Can you work these out from the model? Positions are in its coordinate system, mm. Face numbers are marked on the shaded views. A direction names the side the tool comes from. Give positions to 0.01 mm unless a question says otherwise; leave off trailing zeros. Write each loop counter-clockwise with the first axis right and the second up, starting at its lowest first coordinate (ties: lowest second). Pieces come first, ordered by that corner, then holes.
from build123d import *

# Parameters (mm, degrees)
SKETCH_1_W          = 40
SKETCH_1_H          = 20
EXTRUDE_1_DEPTH     = 3.5
SKETCH_2_W          = 40
SKETCH_2_H          = 20
SKETCH_2_R          = 5.25
EXTRUDE_2_DEPTH     = 1.5
EXTRUDE_3_DEPTH     = 8
SKETCH_4_W          = 40
SKETCH_4_H          = 12
SKETCH_4_R          = 3.5
EXTRUDE_4_DEPTH     = 5
FILLET_1_R          = 1.5
SKETCH_5_R          = 1.75
CUT_EXTRUDE_1_DEPTH = 5
CUT_EXTRUDE_2_DEPTH = 3
CUT_EXTRUDE_3_DEPTH = 3.5
CUT_EXTRUDE_START   = -3.5
SKETCH_8_R          = 5.45
SKETCH_8_R_2        = 5.25
CUT_EXTRUDE_4_DEPTH = 3.5


with BuildPart() as part:
    # 草图1 → 凸台-拉伸1 (new body)
    with BuildSketch(Plane.XY):
        Rectangle(SKETCH_1_W, SKETCH_1_H)
        with BuildLine():
            Line((-9.5, -5.75), (9.5, -5.75))
            ThreePointArc((9.5, -5.75), (11, 0), (9.5, 5.75))
            Line((9.5, 5.75), (-9.5, 5.75))
            ThreePointArc((-9.5, 5.75), (-11, 0), (-9.5, -5.75))
        make_face(mode=Mode.SUBTRACT)
    extrude(amount=EXTRUDE_1_DEPTH)

    # 草图2 → 凸台-拉伸2 (add)
    with BuildSketch(Plane.XY.offset(3.5)):
        Rectangle(SKETCH_2_W, SKETCH_2_H)
        Circle(SKETCH_2_R, mode=Mode.SUBTRACT)
    extrude(amount=EXTRUDE_2_DEPTH)

    # 草图3 → 凸台-拉伸3 (add)
    with BuildSketch(Plane.XY.offset(5)):
        Polygon((-16.560660172, 5.5), (-18.2, 5.5), (-18.2, 3.1), (-20, 3.1), (-20, -3.1), (-18.2, -3.1), (-18.2, -5.5), (-16.560660172, -5.5), (-13.9, -2.839339828), (-13.9, 2.839339828), align=None)
        Polygon((18.2, 3.1), (20, 3.1), (20, -3.1), (18.2, -3.1), (18.2, -5.5), (16.560660172, -5.5), (13.9, -2.839339828), (13.9, 2.839339828), (16.560660172, 5.5), (18.2, 5.5), align=None)
    extrude(amount=-EXTRUDE_3_DEPTH)

    # 草图4 → 凸台-拉伸4 (add)
    with BuildSketch(Plane.XY.offset(5)):
        with Locations((0, 16)):
            Rectangle(SKETCH_4_W, SKETCH_4_H)
        with Locations((-10, 14.64)):
            Circle(SKETCH_4_R, mode=Mode.SUBTRACT)
        with Locations((10, 14.64)):
            Circle(SKETCH_4_R, mode=Mode.SUBTRACT)
    extrude(amount=-EXTRUDE_4_DEPTH)

    # 圆角1
    fillet_1_edges = [part.edges().sort_by_distance(p)[0] for p in [
        (20, 22, 2.5),
        (-20, 22, 2.5),
        (20, -10, 2.5),
        (-20, -10, 2.5),
    ]]
    fillet(fillet_1_edges, radius=FILLET_1_R)

    # 草图5 → 切除-拉伸1 (cut)
    with BuildSketch(Plane.XY.offset(5)):
        with Locations((0, 14.64)):
            Circle(SKETCH_5_R)
    extrude(amount=-CUT_EXTRUDE_1_DEPTH, mode=Mode.SUBTRACT)

    # 草图6 → 切除-拉伸2 (cut)
    with BuildSketch(Plane(origin=(0, 0, -3), x_dir=(-1, 0, 0), z_dir=(0, 0, -1))):
        Polygon((-18.2, 5.5), (-18.2, 3.1), (-20, 3.1), (-20, 2.6), (-19.5, 2.6), (-17.7, 2.6), (-17.7, 5), (-16.767766953, 5), (-14.4, 2.632233047), (-14.4, -2.632233047), (-16.767766953, -5), (-17.7, -5), (-17.7, -2.6), (-19.5, -2.6), (-20, -2.6), (-20, -3.1), (-18.2, -3.1), (-18.2, -5.5), (-16.560660172, -5.5), (-13.9, -2.839339828), (-13.9, 2.839339828), (-16.560660172, 5.5), align=None)
        Polygon((18.2, -5.5), (18.2, -3.1), (20, -3.1), (20, -2.6), (19.5, -2.6), (17.7, -2.6), (17.7, -5), (16.767766953, -5), (14.4, -2.632233047), (14.4, 2.632233047), (16.767766953, 5), (17.7, 5), (17.7, 2.6), (19.5, 2.6), (20, 2.6), (20, 3.1), (18.2, 3.1), (18.2, 5.5), (16.560660172, 5.5), (13.9, 2.839339828), (13.9, -2.839339828), (16.560660172, -5.5), align=None)
    extrude(amount=-CUT_EXTRUDE_2_DEPTH, mode=Mode.SUBTRACT)

    # 草图7 → 切除-拉伸3 (cut)
    with BuildSketch(Plane(origin=(0, 0, 0), x_dir=(-1, 0, 0), z_dir=(0, 0, -1))):
        with BuildLine():
            Line((9.616579756, 5.95), (-9.616579756, 5.95))
            ThreePointArc((-9.616579756, 5.95), (-11.2, 0), (-9.616579756, -5.95))
            Line((-9.616579756, -5.95), (9.616579756, -5.95))
            ThreePointArc((9.616579756, -5.95), (11.2, 0), (9.616579756, 5.95))
        make_face()
    extrude(amount=-CUT_EXTRUDE_3_DEPTH, mode=Mode.SUBTRACT)

    # 草图8 → 切除-拉伸4 (cut)
    with BuildSketch(Plane.XY.offset(5).offset(CUT_EXTRUDE_START)):
        Circle(SKETCH_8_R)
        Circle(SKETCH_8_R_2, mode=Mode.SUBTRACT)
    extrude(amount=CUT_EXTRUDE_4_DEPTH, mode=Mode.SUBTRACT)


solid = part.part
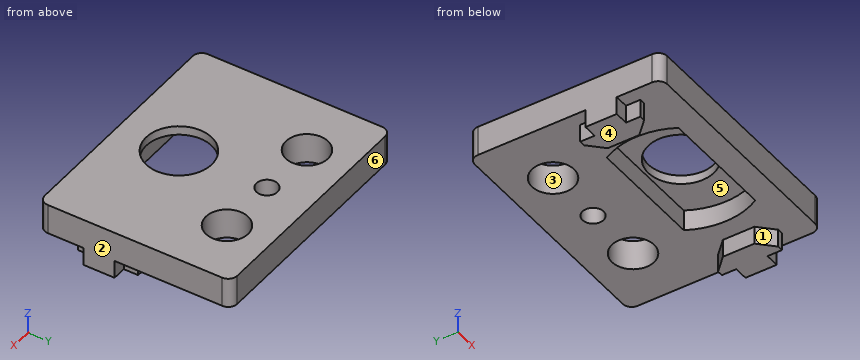
(1) Will these pins go through, and if not, where does the flat tip stop? P1, Ø12.5, axis at x = 0, y = 0, coming from the +Z side; P2, Ø9.5, axis at x = -1.5, y = 1.5, coming from the -Z side; P3, Ø1.9, axis at y = 4, z = -1.5, coming from the -X side; P4, Ø5.5, axis at x = 10, y = 14.64, coming from the -Z side.
Returned:
P1: stops at z = 5
P2: stops at z = 0
P3: stops at x = -17.7
P4: passes through
(2) If I drill on L1, parallel to Y at x = 0, z = 3.6; L2, parallel to Y at x = 0, z = 1.85; L3, parallel to X at y = -1, z = -1.5, over which ranges is the centre line in solid material (lowest first)?
Returned:
L1: y = -10 to -5.45, 5.45 to 12.89, 16.39 to 22
L2: y = -10 to -5.95, 5.95 to 12.89, 16.39 to 22
L3: x = -20 to -14.4, 14.4 to 20
(3) Imagine slicing it at A-A, the plane y = 14.64. Write out the boundary of the cut face in (x, z), plus the area to 4 significant figures.
Returned:
outline: (-20, 0) - (-13.5, 0) - (-13.5, 5) - (-20, 5) - close; (-6.5, 0) - (-1.75, 0) - (-1.75, 5) - (-6.5, 5) - close; (1.75, 0) - (6.5, 0) - (6.5, 5) - (1.75, 5) - close; (13.5, 0) - (20, 0) - (20, 5) - (13.5, 5) - close
area: 112.5 mm2
(4) Imagine slicing it at D-D, the plane y = 0. Write out the boundary of the cut face in (x, z).
Returned:
outline: (-20, -3) - (-14.4, -3) - (-14.4, 0) - (-11.2, 0) - (-11.2, 3.5) - (-5.45, 3.5) - (-5.45, 5) - (-20, 5) - close; (5.45, 3.5) - (11.2, 3.5) - (11.2, 0) - (14.4, 0) - (14.4, -3) - (20, -3) - (20, 5) - (5.45, 5) - close
(5) For the marked faces 5 and 6, which set-ups out of +Z, -Z, +X, -X, +Y, -Y let a thin tool reach every point of the face, with its end or its side?
Returned:
face 5: -Z
face 6: +Z, -Z, +X, -X, +Y
(6) If we mould it in two halves opening along X, with no side actions, what happens to the marked faces 1, 2, 3 and 4? For each: +X half, -X half, draft (parallel to the pull), parting line (faces both ways), or undercut.
Returned:
face 1: undercut
face 2: +X half
face 3: undercut
face 4: draft
(7) Imagine slicing it at B-B, the plane x = 0. Write out the boundary of the cut face in (y, z).
Returned:
outline: (-10, 0) - (-5.95, 0) - (-5.95, 3.5) - (-5.45, 3.5) - (-5.45, 5) - (-10, 5) - close; (5.45, 3.5) - (5.95, 3.5) - (5.95, 0) - (12.89, 0) - (12.89, 5) - (5.45, 5) - close; (16.39, 0) - (22, 0) - (22, 5) - (16.39, 5) - close
(8) Imagine slicing it at C-C, the plane z = -1.5. Write out the boundary of the cut face in (x, y), plus the area to 3 significant figures.
Returned:
outline: (-20, -2.6) - (-17.7, -2.6) - (-17.7, -5) - (-16.77, -5) - (-14.4, -2.63) - (-14.4, 2.63) - (-16.77, 5) - (-17.7, 5) - (-17.7, 2.6) - (-20, 2.6) - close; (14.4, -2.63) - (16.77, -5) - (17.7, -5) - (17.7, -2.6) - (20, -2.6) - (20, 2.6) - (17.7, 2.6) - (17.7, 5) - (16.77, 5) - (14.4, 2.63) - close
area: 78.7 mm2
